Work out the finished part from the listing and answer in its coordinate system (mm). A direction names the side the tool comes from. Give positions to 0.01 mm unless a question says otherwise; leave off trailing zeros. Write each loop counter-clockwise with the first axis right and the second up, starting at its lowest first coordinate (ties: lowest second). Pieces come first, ordered by that corner, then holes. Notation, with made-up numbers: (70, -10.5) -> (128, -10.5) arc R19 cw to (128, 8.5) -> close; hole circle Ø7 at (-25, 56.25). An arc over 180 degrees is marked (long way). Write item = value, one per line. Start each with the question number.
from build123d import *

# Parameters (mm, degrees)
SKETCH_1_R             = 5.25
SM_BASE_FLANGE_1_DEPTH = 4


# Sheet-metal steps are written as plain solids
with BuildPart() as part:
    # Sketch 1 → Базовая кромка1 (new body)
    with BuildSketch(Plane(origin=(0, 0, 0), x_dir=(1, 0, 0), z_dir=(0, 1, 0))):
        Polygon((39.244426356, -13.081475452), (-13.081475452, 39.244426356), (-13.081475452, 54.244426356), (-45.40737726, 54.244426356), (-45.40737726, 19.244426356), (19.244426356, -45.40737726), (54.244426356, -45.40737726), (54.244426356, -13.081475452), align=None)
        with Locations(Location((-13.081475452, 13.081475452, 0), (0, 0, 270))):
            Circle(SKETCH_1_R, mode=Mode.SUBTRACT)
        with Locations(Location((13.081475452, -13.081475452, 0), (0, 0, 90))):
            Circle(SKETCH_1_R, mode=Mode.SUBTRACT)
    extrude(amount=-SM_BASE_FLANGE_1_DEPTH)


solid = part.part
(1) For faces 1 (the flat face through (4, 0, -5)), 2 (the flat face through (-13.081, -2, -47)), determine the directions among +Z, -Z, +X, -X, +Y, -Y from which every point of the face is accessible in a straight line to the end or side of a thin tool.
(2) Each of these flat-tipped pins is pushed along its axis until it touches: pin 1 (2 mm diameter, centred on x = 43, y = -1.5, fed in from -Z); pin 2 (2 mm diameter, centred on x = -2, y = -1.5, fed in from +Z); pin 3 (1 mm diameter, centred on y = -2, z = -43.5, fed in from +X). Where does it stop, or does it pass through?
(3) A cutting plane is placed at C-C, the plane z = -42.5. Write down the section's boundary in (x, y), then the cut area to 3 significant figures.
(4) A cutting plane is placed at B-B, the plane z = -10. Write down the section's boundary in (x, y), then the cut area to 3 significant figures.
(5) Determine the mould class of faces 3 (the flat face through (-45.407, -2, -37)), 4 (the flat face through (-29, -2, -54.244)), 5 (the cylindrical face through (-17.74, -1.97, -10.66)) for opening direction X: pulls with the +X half, pulls with the -X half, needs draft (parallel to the pull), parting line crosses it, or undercut.
(6) A cutting plane is placed at A-A, the plane y = -2.55. Write down the section's boundary in (x, z).
(7) A cutting plane is placed at D-D, the plane x = -4.5. Write down the section's boundary in (y, z), then the cut area to 3 significant figures.
(8) Find the intervals of material crossed by line 1 along X through (y, z) = (-2.75, -49); line 2 along Z through (x, y) = (13, -1.85); line 3 along X through (y, z) = (-0.5, -9), in increasing order.
Results list:
q1.face_1 = +Z, -Z, +X, -X, +Y
q1.face_2 = -Z, +X, +Y, -Y
q2.pin_1 = 13.08
q2.pin_2 = 25.16
q2.pin_3 = -13.08
q3.outline = (-45.41, -4) -> (-13.08, -4) -> (-13.08, 0) -> (-45.41, 0) -> close
q3.area = 129 mm²
q4.outline = (-36.16, -4) -> (-17.33, -4) -> (-17.33, 0) -> (-36.16, 0) -> close; (-8.83, -4) -> (16.16, -4) -> (16.16, 0) -> (-8.83, 0) -> close
q4.area = 175 mm²
q5.face_3 = pulls with the -X half
q5.face_4 = needs draft
q5.face_5 = undercut
q6.outline = (-45.41, -54.24) -> (-13.08, -54.24) -> (-13.08, -39.24) -> (39.24, 13.08) -> (54.24, 13.08) -> (54.24, 45.41) -> (19.24, 45.41) -> (-45.41, -19.24) -> close; hole circle Ø10.5 at (-13.08, -13.08); hole circle Ø10.5 at (13.08, 13.08)
q7.outline = (-4, -30.66) -> (0, -30.66) -> (0, 21.66) -> (-4, 21.66) -> close
q7.area = 209 mm²
q8.line_1 = -45.41 to -13.08
q8.line_2 = -13.16 to 7.83, 18.33 to 39.16
q8.line_3 = -35.16 to -16.38, -9.78 to 17.16
